Input: part model. Units: mm. Frame: model coordinates. Face numbers are marked on the shaded views. Coordinates: 2 decimals unless noted, no trailing zeros. Write each loop counter-clockwise with the first axis right and the second up, starting at its lowest first coordinate (ties: lowest second). Pieces come first, ordered by that corner, then holes. Notation, with made-up numbers: M 89.25,9.5 L 129.25,9.5 A21 cw 129.25,19.5 Z; hole C -22.75,-22 d1. An arc over 180 degrees is marked long. Use one line per item in the form item = value.
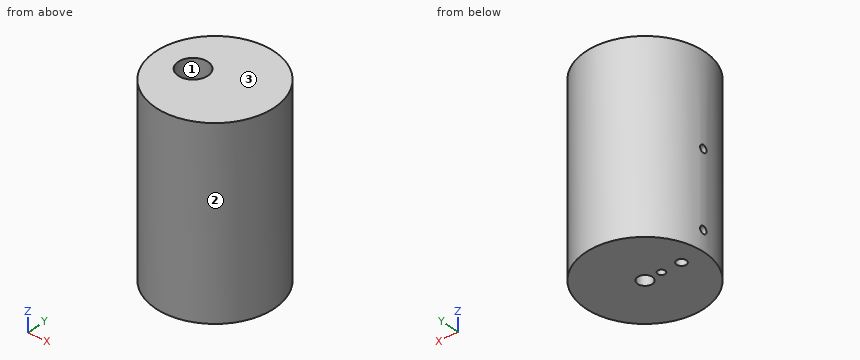
from build123d import *

# Parameters (mm, degrees)
SKETCH1_R           = 40
BOSS_EXTRUDE1_DEPTH = 125
SKETCH9_R           = 16
CUT_EXTRUDE3_DEPTH  = 38.79
SKETCH11_R          = 2.5
CUT_EXTRUDE5_DEPTH  = 10
SKETCH10_R          = 5
CUT_EXTRUDE4_DEPTH  = 38.5
SKETCH12_R          = 2.5
CUT_EXTRUDE7_DEPTH  = 44
SKETCH13_R          = 2.5
CUT_EXTRUDE8_DEPTH  = 64
SKETCH14_R          = 3.25
CUT_EXTRUDE9_DEPTH  = 20
SKETCH16_R          = 2.5
CUT_EXTRUDE10_DEPTH = 36
SKETCH18_R          = 2.5
CUT_EXTRUDE11_DEPTH = 29
SKETCH21_R          = 10
CUT_EXTRUDE12_DEPTH = 40
SKETCH22_R          = 2.5
CUT_EXTRUDE13_DEPTH = 21


with BuildPart() as part:
    # Sketch1 → Boss-Extrude1 (new body)
    with BuildSketch(Plane.XY):
        Circle(SKETCH1_R)
    extrude(amount=BOSS_EXTRUDE1_DEPTH)

    # Sketch9 → Cut-Extrude3 (cut)
    with BuildSketch(Plane.XY.offset(18.19)):
        Circle(SKETCH9_R)
    extrude(amount=CUT_EXTRUDE3_DEPTH, mode=Mode.SUBTRACT)

    # Sketch11 → Cut-Extrude5 (cut)
    with BuildSketch(Plane(origin=(0, 0, 56.98), x_dir=(-1, 0, 0), z_dir=(0, 0, -1))):
        Circle(SKETCH11_R)
    extrude(amount=-CUT_EXTRUDE5_DEPTH, mode=Mode.SUBTRACT)

    # Sketch10 → Cut-Extrude4 (cut)
    with BuildSketch(Plane.XY):
        Circle(SKETCH10_R)
    extrude(amount=CUT_EXTRUDE4_DEPTH, mode=Mode.SUBTRACT)

    # Sketch12 → Cut-Extrude7 (cut)
    with BuildSketch(Plane(origin=(0, 0, 0), x_dir=(0, 0, -1), z_dir=(1, 0, 0))):
        with Locations(Location((-64, 0, 0), (0, 0, 180))):
            Circle(SKETCH12_R)
    extrude(amount=-CUT_EXTRUDE7_DEPTH, mode=Mode.SUBTRACT)

    # Sketch13 → Cut-Extrude8 (cut)
    with BuildSketch(Plane(origin=(0, 0, 0), x_dir=(-1, 0, 0), z_dir=(0, 0, -1))):
        with Locations((25, 0)):
            Circle(SKETCH13_R)
    extrude(amount=-CUT_EXTRUDE8_DEPTH, mode=Mode.SUBTRACT)

    # Sketch14 → Cut-Extrude9 (cut)
    with BuildSketch(Plane(origin=(0, 0, 0), x_dir=(-1, 0, 0), z_dir=(0, 0, -1))):
        with Locations((25, 0)):
            Circle(SKETCH14_R)
    extrude(amount=-CUT_EXTRUDE9_DEPTH, mode=Mode.SUBTRACT)

    # Sketch16 → Cut-Extrude10 (cut)
    with BuildSketch(Plane(origin=(0, 0, 0), x_dir=(-1, 0, 0), z_dir=(0, 0, -1))):
        with Locations((11.221670406, 0)):
            Circle(SKETCH16_R)
    extrude(amount=-CUT_EXTRUDE10_DEPTH, mode=Mode.SUBTRACT)

    # Sketch18 → Cut-Extrude11 (cut)
    with BuildSketch(Plane(origin=(-40, 0, 0), x_dir=(0, 0, -1), z_dir=(1, 0, 0))):
        with Locations(Location((-13.5, 0, 0), (0, 0, 180))):
            Circle(SKETCH18_R)
    extrude(amount=CUT_EXTRUDE11_DEPTH, mode=Mode.SUBTRACT)

    # Sketch21 → Cut-Extrude12 (cut)
    with BuildSketch(Plane.XY.offset(125)):
        with Locations((-15, 0)):
            Circle(SKETCH21_R)
    extrude(amount=-CUT_EXTRUDE12_DEPTH, mode=Mode.SUBTRACT)

    # Sketch22 → Cut-Extrude13 (cut)
    with BuildSketch(Plane.XY.offset(85)):
        with Locations((-15, 0)):
            Circle(SKETCH22_R)
    extrude(amount=-CUT_EXTRUDE13_DEPTH, mode=Mode.SUBTRACT)


solid = part.part
(1) Section query C-C on z = 94. Return the cut outline in (x, y).
Computed:
outline = C 0,0 d80; hole C -15,0 d20
(2) Section query A-A on y = 0. State how many separate pieces and enclosed holes the cut face has, plus the area to 3 significant figures.
Computed:
separate_pieces = 7
enclosed_holes = 0
area = 6,920 mm^2
(3) Pull-direction query (Y, two-part tool) for the marked faces 1, 2 and 3; classes: pulls with the +Y half, pulls with the -Y half, needs draft (parallel to the pull), parting line crosses it, or undercut.
Computed:
face_1 = undercut
face_2 = parting line crosses it
face_3 = needs draft
(4) First-contact query: pin 1 Ø12 at (y, z) = (-9.5, 47) entering from -X; pin 2 Ø10 at (y, z) = (-16.5, 87.5) entering from +X; pin 3 Ø4 at (x, y) = (-15, 0) entering from +Z. Flat tips, straight axial feed; report the tip coordinate or a pass-through.
Computed:
pin_1 = -39.85
pin_2 = 38.31
pin_3 = 62.5
(5) Section query D-D on y = -30. Return the cut outline in (x, z), plus the area to 3 significant figures.
Computed:
outline = M -26.46,0 L 26.46,0 L 26.46,125 L -26.46,125 Z
area = 6,610 mm^2
(6) Line query: probe 1 along Z at (x, y) = (-21.5, -1); probe 2 along Y at (x, z) = (-25, 5); probe 3 along Y at (x, z) = (0, 45). Output: solid intervals per line, ascending.
Computed:
probe_1 = 0 to 11.21, 15.79 to 61.71, 66.29 to 85
probe_2 = -31.22 to -3.25, 3.25 to 31.22
probe_3 = -40 to -16, 16 to 40
(7) Section query B-B on z = 35. Return the cut outline in (x, y).
Computed:
outline = C 0,0 d80; hole C -25,0 d5; hole C 0,0 d32
